Autodesk Inventor part; units mm, degrees
ref_plane "YZ Plane" through (0, 0, 0) normal (1, 0, 0) x (0, 1, 0)
ref_plane "XZ Plane" through (0, 0, 0) normal (0, 1, 0) x (-1, 0, 0)
ref_plane "XY Plane" through (0, 0, 0) normal (0, 0, 1) x (1, 0, 0)
sketch "스케치1" plane through (0, 0, 0) normal (0, 0, 1) x (1, 0, 0)
  circle A0 centre (0, 0) radius 270
  circle A1 centre (0, 0) radius 165
  dimension "d0" = 540
  dimension "d1" = 330
extrude "돌출1" add sketch "스케치1" along normal mid plane 175
extrude "돌출2" add sketch "스케치1" along normal mid plane 140 contours A1
fillet "모깎기1" radius 4 2 edges at (-165, 0, 87.5) (-165, 0, 70)
fillet "모깎기2" radius 40 2 edges at (-270, 0, 87.5) (-270, 0, -87.5)
sketch "스케치2" plane through (0, 0, 0) normal (0, 0, 1) x (1, 0, 0)
  circle A0 centre (0, 0) radius 25
  circle A1 centre (0, 47.0427) radius 7.5
  circle A2 centre (-47.0427, 0) radius 7.5
  circle A3 centre (0, -47.0427) radius 7.5
  circle A4 centre (47.0427, 0) radius 7.5
  dimension "d8" = 50
  dimension "d9" = 15
  dimension "d12" = 360
extrude "돌출3" add sketch "스케치2" along normal mid plane 150 contours A0
extrude "돌출4" cut sketch "스케치2" along normal mid plane 150 contours A1 | A2 | A3 | A4
sketch "스케치4" plane through (0, 0, 0) normal (1, 0, 0) x (0, 1, 0)
  line L0 (270, -47.5) -> (270, 47.5)
  line L1 (270, 35.3814) -> (267.8692, 35.3814)
  line L2 (267.8692, 35.3814) -> (267.8692, 25.3814)
  line L3 (267.8692, 25.3814) -> (270, 25.3814)
  line L4 (270, 16.4038) -> (267.8692, 16.4038)
  line L5 (267.8692, 16.4038) -> (267.8692, 6.4038)
  line L6 (267.8692, 6.4038) -> (270, 6.4038)
  line L7 (280.9878, 0) -> (263.4352, 0)
  line L8 (270, -35.3814) -> (267.8692, -35.3814)
  line L9 (267.8692, -35.3814) -> (267.8692, -25.3814)
  line L10 (267.8692, -25.3814) -> (270, -25.3814)
  line L11 (267.8692, -6.4038) -> (270, -6.4038)
  line L12 (267.8692, -16.4038) -> (267.8692, -6.4038)
  line L13 (270, -16.4038) -> (267.8692, -16.4038)
  line L14 (0, 108.3744) -> (0, -123.7727) construction
  point P0 (0, 0)
  dimension "d20" = 10
  dimension "d21" = 10
revolve "회전1" cut sketch "스케치4" angle 360 about axis through (0, 0, 108.3744) along (0, 0, -1)
sketch "스케치5" plane through (0, 0, 70) normal (0, 0, 1) x (1, 0, 0)
  circle A0 centre (0, 0) radius 157.111
extrude "돌출5" cut sketch "스케치5" along normal blind 50 and the other way blind 100
sketch "스케치8" plane through (0, 0, -30) normal (0, 0, 1) x (1, 0, 0)
  circle A0 centre (0, 0) radius 7.5
  dimension "d31" = 15
extrude "돌출6" add sketch "스케치8" along normal blind 10
properties part number "wheel" material "고무"
Can you work these out from the model? Positions are in its coordinate system, mm. A direction names the side the tool comes from. Coordinates: 2 decimals unless noted, no trailing zeros. Write each loop counter-clockwise with the first axis right and the second up, starting at its lowest first coordinate (ties: lowest second). Pieces come first, ordered by that corner, then holes. Notation, with made-up numbers: (-19.75, 26.25) - (29.25, 26.25) arc R26 cw to (29.25, 54.25) - close; hole circle Ø11 at (48.5, -6). An arc over 180 degrees is marked (long way). Return JSON: item names as keys, results as strings.
Q1. Thinking about a two-plate mould opening in Y: for faces 1 (the cylindrical face through (-80.46, 255.5, -11.33)), 2 (the flat face through (0, 0, -75)), which applies, +Y half, -Y half, draft (parallel to the pull), parting line (faces both ways), or undercut?
Computed values:
{"face 1": "parting line", "face 2": "undercut"}
Q2. I'm going to push flat-ended pins straight in: pin 1 Ø10 at (x, y) = (-20.5, 17.5) entering from -Z; pin 2 Ø17 at (x, y) = (-47.04, 0) entering from +Z; pin 3 Ø24 at (x, y) = (0, -47.04) entering from -Z. Where does each tip first touch, or does it pass through?
Computed values:
{"pin 1": "stops at z = -75", "pin 2": "stops at z = -30", "pin 3": "stops at z = -70"}
Q3. Please list where these lines run through material, in increasing order: L1, parallel to Y at x = 0, z = -45; L2, parallel to Y at x = 6.5, z = -53.5; L3, parallel to Z at x = -118, y = -32. Write a range as from..to.
Computed values:
{"L1": "y = -270..-54.54, -39.54..39.54, 54.54..270", "L2": "y = -269.47..-50.78, -43.3..43.3, 50.78..269.47", "L3": "z = -70..-30"}
Q4. If we section it at A-A (y = 0): Count the separate pieces of the cut face and the enclosed holes in it, then the cut area to 3 significant figures.
Computed values:
{"separate pieces": "3", "enclosed holes": "0", "area": "49,200 mm2"}
Q5. On a 3-axis mill with a long thin cutter (end or side, diameter ignored), from which of +Z, -Z, +X, -X, +Y, -Y can I reach the whole of each face in a straight line? I mean faces 3 (the cylindrical face through (80.46, 255.5, 30.31)), 4 (the flat face through (-2, -34, -70)), 5 (the flat face through (35, -154, 70)), 6 (the cylindrical face through (39.55, 0.33, -49.72)). Say none if no direction works.
Computed values:
{"face 3": "none", "face 4": "-Z", "face 5": "+Z", "face 6": "+Z, -Z"}
Q6. If we section it at C-C (z = 61.5): Please give me the cut outline in (x, y), then the cut area to 3 significant figures.
Computed values:
{"outline": "circle Ø534.94 at (0, 0); hole circle Ø314.22 at (0, 0)", "area": "147,000 mm2"}
